The model under review builds one solid part; all positions refer to its coordinate system, in mm. A direction names the side the tool comes from. Round coordinates to 2 decimals unless told otherwise and drop trailing zeros. Order: outer loops, then holes, each group sorted by start corner. A loop starts at its lowest first (then second) coordinate and runs counter-clockwise, first axis right, second up. Notation, with made-up numbers: M -9,72 L 25,72 A19 ccw 25,91 Z; hole C 31.25,20.25 d6. An arc over 180 degrees is marked long. Answer as a JSON object with one key per item and string values. Group by question number.
1) For faces 4 (the flat face through (8.45, -6.5, 1.2)), 5 (the flat face through (7.35, -8, 1)), 6 (the cylindrical face through (-5.347, -0.158, 4.986)), 7 (the flat face through (9, -5.5, 1)), list the 3-axis set-ups (+Z, -Z, +X, -X, +Y, -Y) from which the entire face can be reached by the end or side of a thin tool; tool diameter is ignored.
2) Consider section B-B, the plane y = -10.5. Write out the cut boundary in (x, z), then the cut area to 3 significant figures.
3) Consider section D-D, the plane z = 4.95. Write out the cut boundary in (x, y), then the cut area to 3 significant figures.
4) Insertion check: pin 1 Ø1.8 at (x, z) = (-1.5, 1.5) entering from -Y; pin 2 Ø1.8 at (y, z) = (-1, 1.5) entering from -X; pin 3 Ø1.2 at (y, z) = (-8, 1.5) entering from +X. Each pin has a flat end and moves straight along its axis. Give the tip position at first contact, or say it passes through.
5) Consider section A-A, the plane x = 9.9. Write out the cut boundary in (y, z), then the cut area to 3 significant figures.
6) The part is to be moulded in two halves that separate along X. For faces 1 (the cylindrical face through (9.163, 9.824, 0.246)), 2 (the flat face through (8, -9, 1)), 3 (the flat face through (9.45, -6, 1)), say which applies: +X half, -X half, draft (parallel to the pull), parting line (faces both ways), or undercut.
7) Consider section C-C, the plane y = -1.5. Write out the cut boundary in (x, z).
8) To check wall thickness, follow line 1 (Y direction, x = -2.6, z = 0.35); line 2 (X direction, y = -2.25, z = 0.75); line 3 (Z direction, x = 4.5, y = 4.25). State the ranges of each line that lie inside material, in increasing order.
Autodesk Inventor part; units mm, degrees
ref_plane "YZ Plane" through (0, 0, 0) normal (1, 0, 0) x (0, 1, 0)
ref_plane "XZ Plane" through (0, 0, 0) normal (0, 1, 0) x (-1, 0, 0)
ref_plane "XY Plane" through (0, 0, 0) normal (0, 0, 1) x (1, 0, 0)
sketch "Sketch1" plane through (0, 0, 0) normal (0, 0, 1) x (1, 0, 0)
  line L0 (-11.95, 12.5) -> (11.95, 12.5)
  line L1 (11.95, 12.5) -> (11.95, -12.5)
  line L2 (11.95, -12.5) -> (-11.95, -12.5)
  line L3 (-11.95, -12.5) -> (-11.95, 12.5)
  line L4 (-11.95, 12.5) -> (11.95, -12.5) construction
  line L5 (11.95, 12.5) -> (-11.95, -12.5) construction
  circle A0 centre (9.9, -10.5) radius 1
  circle A1 centre (-2.6, -10.5) radius 1
  line L6 (11.5332, -10.5) -> (-16.0268, -10.5) construction
  line L7 (9.9, -13.3661) -> (9.9, 11.2852) construction
  line L8 (11.2708, 10.5) -> (-4.8598, 10.5) construction
  circle A2 centre (9.9, 10.5) radius 1
  line L9 (-2.6, -15.3332) -> (-2.6, 11.9823) construction
  circle A3 centre (-2.6, 10.5) radius 1
  point P0 (0, 0)
  dimension "d0" = 23.9
  dimension "d1" = 25
  dimension "d2" = 2
  dimension "d3" = 21.85
  dimension "d5" = 2
  dimension "d6" = 9.35
  dimension "d7" = 2
  dimension "d8" = 23
  dimension "d9" = 2
  dimension "d10" = 2
extrude "Extrusion1" add sketch "Sketch1" along normal blind 0.5
sketch "Sketch2" plane through (0, 0, 0.5) normal (0, 0, 1) x (1, 0, 0)
  line L0 (-16.73, 0) -> (16.73, 0) construction
  line L1 (-5.95, 4.2) -> (2.45, 4.2)
  line L2 (2.45, 4.2) -> (2.45, -4.2)
  line L3 (2.45, -4.2) -> (-5.95, -4.2)
  line L4 (-5.95, -4.2) -> (-5.95, 4.2)
  line L5 (-5.95, 4.2) -> (2.45, -4.2) construction
  line L6 (2.45, 4.2) -> (-5.95, -4.2) construction
  line L7 (-11.95, 12.5) -> (-11.95, -12.5)
  point P0 (0, 0)
  point P1 (-1.75, 0)
  dimension "d13" = 8.4
  dimension "d14" = 8.4
  dimension "d15" = 6
extrude "Extrusion2" add sketch "Sketch2" along normal blind 3.5
sketch "Sketch3" plane through (0, 0, 4) normal (0, 0, 1) x (1, 0, 0)
  line L0 (-5.95, 4.2) -> (2.45, 4.2) construction
  line L1 (-5.95, 4.2) -> (2.45, -4.2) construction
  line L2 (-5.95, -4.2) -> (2.45, -4.2) construction
  line L3 (2.45, 4.2) -> (-5.95, -4.2) construction
  circle A0 centre (-1.75, 0) radius 3.6
  point P0 (0, 0)
  dimension "d18" = 7.2
extrude "Extrusion3" add sketch "Sketch3" along normal blind 2
sketch "Sketch4" plane through (0, 0, 0.5) normal (0, 0, 1) x (1, 0, 0)
  line L0 (7.35, -7) -> (8.35, -7)
  line L1 (8.35, -7) -> (8.35, -9)
  line L2 (8.35, -9) -> (7.35, -9)
  line L3 (7.35, -9) -> (7.35, -7)
  line L4 (8.45, -5.5) -> (9.45, -5.5)
  line L5 (9.45, -5.5) -> (9.45, -7.5)
  line L6 (9.45, -7.5) -> (8.45, -7.5)
  line L7 (8.45, -7.5) -> (8.45, -5.5)
  line L8 (-11.95, -12.5) -> (11.95, -12.5)
  line L9 (11.95, -12.5) -> (11.95, 12.5)
  point P0 (0, 0)
  dimension "d21" = 3.5
  dimension "d22" = 1
  dimension "d23" = 2
  dimension "d25" = 2.5
  dimension "d26" = 1
  dimension "d27" = 2
  dimension "d28" = 5
  dimension "d31" = 0.1
extrude "Extrusion4" add sketch "Sketch4" along normal blind 1.5
properties part number "Board"
Results list:
{
 "1": {"face 4": "+Z, +Y, -Y", "face 5": "+Z, -X, +Y, -Y", "face 6": "+Z", "face 7": "+Z, +X, -X, +Y"},
 "2": {"outline": "M -11.95,0 L -3.6,0 L -3.6,0.5 L -11.95,0.5 Z; M -1.6,0 L 8.9,0 L 8.9,0.5 L -1.6,0.5 Z; M 10.9,0 L 11.95,0 L 11.95,0.5 L 10.9,0.5 Z", "area": "9.95 mm^2"},
 "3": {"outline": "C -1.75,0 d7.2", "area": "40.7 mm^2"},
 "4": {"pin 1": "y = -4.2", "pin 2": "x = -5.95", "pin 3": "x = 9.45"},
 "5": {"outline": "M -12.5,0 L -11.5,0 L -11.5,0.5 L -12.5,0.5 Z; M -9.5,0 L 9.5,0 L 9.5,0.5 L -9.5,0.5 Z; M 11.5,0 L 12.5,0 L 12.5,0.5 L 11.5,0.5 Z", "area": "10.5 mm^2"},
 "6": {"face 1": "undercut", "face 2": "draft", "face 3": "+X half"},
 "7": {"outline": "M -11.95,0 L 11.95,0 L 11.95,0.5 L 2.45,0.5 L 2.45,4 L 1.52,4 L 1.52,6 L -5.02,6 L -5.02,4 L -5.95,4 L -5.95,0.5 L -11.95,0.5 Z"},
 "8": {"line 1": "-12.5 to -11.5, -9.5 to 9.5, 11.5 to 12.5", "line 2": "-5.95 to 2.45", "line 3": "0 to 0.5"}
}
